Input: part model. Units: mm. Frame: model coordinates. Face numbers are marked on the shaded views. A direction names the side the tool comes from. Give positions to 0.01 mm unless a question says otherwise; leave off trailing zeros. Order: outer loops, then holes, each group sorted by start corner. A loop starts at its lowest first (then second) coordinate and runs counter-clockwise, first axis right, second up. Notation, with made-up numbers: (-5.5, -39.5) - (26.5, -39.5) arc R32 ccw to (26.5, -5.5) - close; hole circle Ø1 at (-1.5, -38.75). An arc over 180 degrees is marked (long way). Answer in a Markdown table with one row per item. Add a question column.
1. Section query C-C on y = -4.75. Return loops of the section in (x, z).
2. Contact query for flat-ended pins moving along their axis: pin 1 (6 mm diameter, centred on x = 42, y = -5.5, fed in from -Z); pin 2 (2.5 mm diameter, centred on x = 0, z = 0, fed in from -Y); pin 3 (3 mm diameter, centred on x = 17.5, y = -5, fed in from -Z); pin 4 (1.9 mm diameter, centred on x = 28, y = -3.5, fed in from +Z). Output: stop coordinate, or through.
3. Access query for the marked faces 1, 2 and 3. Directions: +Z, -Z, +X, -X, +Y, -Y. A direction counts if a zero-diameter tool reaches every point of the face in a straight line with its end or side. Return the directions, or none.
4. Section query A-A on x = -50. Return loops of the section in (y, z), and give its area (3 significant figures).
5. Section query B-B on x = -13. Return loops of the section in (y, z).
6. Ray query, line 1 (X direction, y = -1, z = -1.25); line 2 (X direction, y = -5.75, z = 0.1); line 3 (Z direction, x = -50, y = -0.7). Return the intervals inside material, ascending. Write a range as [from, to].
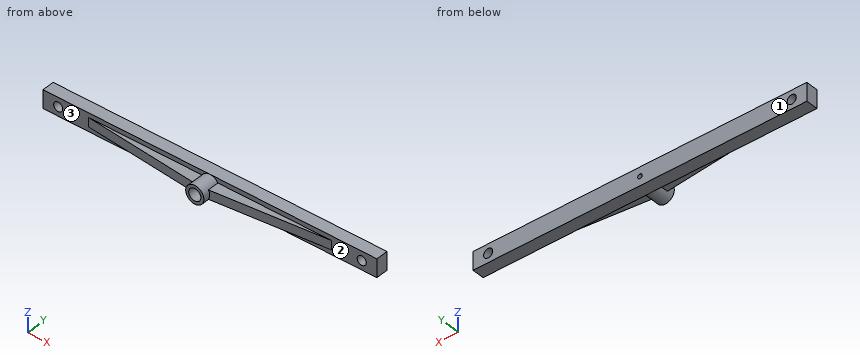
```python
from build123d import *

# Parameters (mm, degrees)
SKETCH1_W                  = 110
SKETCH1_H                  = 4
BOSS_EXTRUDE1_DEPTH        = 3
BOSS_EXTRUDE2_DEPTH        = 1.5
F_3_0_3_DIAMETER_HOLE1_D   = 3
SKETCH5_R                  = 3
BOSS_EXTRUDE3_DEPTH        = 6
F_1_5_1_5_DIAMETER_HOLE1_D = 1.5
SKETCH8_R                  = 2
CUT_EXTRUDE1_DEPTH         = 6


with BuildPart() as part:
    # Sketch1 → Boss-Extrude1 (new, symmetric)
    with BuildSketch(Plane.XY):
        Rectangle(SKETCH1_W, SKETCH1_H)
    extrude(amount=BOSS_EXTRUDE1_DEPTH, both=True)

    # Sketch2 → Boss-Extrude2 (add, symmetric)
    with BuildSketch(Plane.XY):
        Polygon((-40, -2), (0, -6), (40, -2), align=None)
    extrude(amount=BOSS_EXTRUDE2_DEPTH, both=True)

    # Ø3.0 (3) Diameter Hole1 (through all)
    with Locations(Plane(origin=(0, 2, 0), x_dir=(1, 0, 0), z_dir=(0, 1, 0))):
        with Locations((-50, 0), (50, 0)):
            Hole(F_3_0_3_DIAMETER_HOLE1_D / 2)

    # Sketch5 → Boss-Extrude3 (add)
    with BuildSketch(Plane.XZ.offset(2)):
        with Locations(Location((0, 0, 0), (0, 0, 150))):
            Circle(SKETCH5_R)
    extrude(amount=BOSS_EXTRUDE3_DEPTH)

    # Ø1.5 (1.5) Diameter Hole1 (through all)
    with Locations(Plane(origin=(0, -8, 0), x_dir=(-1, 0, 0), z_dir=(0, -1, 0))):
        with Locations((0, 0)):
            Hole(F_1_5_1_5_DIAMETER_HOLE1_D / 2)

    # Sketch8 → Cut-Extrude1 (cut)
    with BuildSketch(Plane.XZ.offset(8)):
        Circle(SKETCH8_R)
    extrude(amount=-CUT_EXTRUDE1_DEPTH, mode=Mode.SUBTRACT)


solid = part.part
```
Answer:
| question | item | result |
|---|---|---|
| 1 | outline | (-12.5, -1.5) - (-2.6, -1.5) arc R3 ccw to (2.6, -1.5) - (12.5, -1.5) - (12.5, 1.5) - (2.6, 1.5) arc R3 ccw to (-2.6, 1.5) - (-12.5, 1.5) - close; hole circle Ø4 at (0, 0) |
| 2 | pin 1 | passes through |
| 2 | pin 2 | stops at y = -2 |
| 2 | pin 3 | stops at z = -1.5 |
| 2 | pin 4 | stops at z = 1.5 |
| 3 | face 1 | +Z, -Z, +X, -X, +Y |
| 3 | face 2 | +X, -Y |
| 3 | face 3 | -X, -Y |
| 4 | outline | (-2, -3) - (2, -3) - (2, -1.5) - (-2, -1.5) - close; (-2, 1.5) - (2, 1.5) - (2, 3) - (-2, 3) - close |
| 4 | area | 12.0 mm² |
| 5 | outline | (-4.7, -1.5) - (-2, -1.5) - (-2, -3) - (2, -3) - (2, 3) - (-2, 3) - (-2, 1.5) - (-4.7, 1.5) - close |
| 6 | line 1 | x = [-55, -50.83], [-49.17, 49.17], [50.83, 55] |
| 6 | line 2 | x = [-3, -2], [2, 3] |
| 6 | line 3 | z = [-3, -1.5], [1.5, 3] |
